from build123d import *

# Parameters (mm, degrees)
F0_W     = 50.8
F0_H     = 50.8
F0_W_2   = 41.275
F0_H_2   = 41.275
F1_DEPTH = 171.45
F2_R     = 5.08
F3_R     = 5.08


with BuildPart() as f1:
    # F0 (on Front) → F1 (new body, symmetric)
    with BuildSketch(Plane.XZ):
        Rectangle(F0_W, F0_H)
        Rectangle(F0_W_2, F0_H_2, mode=Mode.SUBTRACT)
    extrude(amount=F1_DEPTH, both=True)

    # F2
    f2_edges = [f1.edges().sort_by_distance(p)[0] for p in [
        (-20.6375, 0, 20.6375),
        (-25.4, 0, -25.4),
        (25.4, 0, -25.4),
        (20.6375, 0, 20.6375),
        (25.4, 0, 25.4),
        (-25.4, 0, 25.4),
    ]]
    fillet(f2_edges, radius=F2_R)

    # F3
    f3_edges = [f1.edges().sort_by_distance(p)[0] for p in [
        (-20.6375, 0, -20.6375),
        (20.6375, 0, -20.6375),
    ]]
    fillet(f3_edges, radius=F3_R)


solid = f1.part
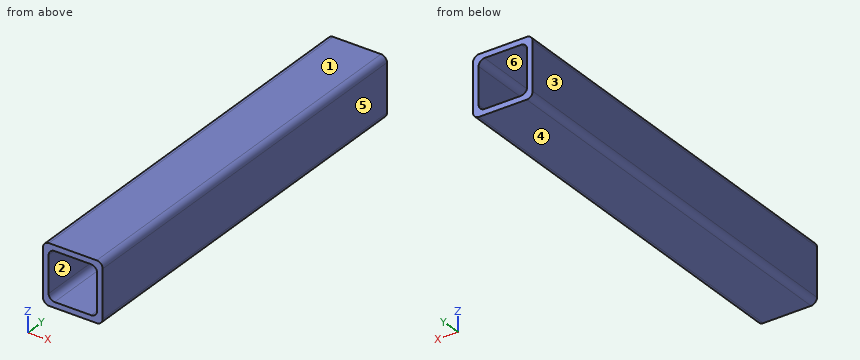
Geometry: final body of the model. Coordinates: model frame, mm. Face numbers are marked on the shaded views. A direction names the side the tool comes from. Give positions to 0.01 mm unless a question says otherwise; leave off trailing zeros. Write each loop counter-clockwise with the first axis right and the second up, starting at its lowest first coordinate (ties: lowest second). Pieces come first, ordered by that corner, then holes. Notation, with made-up numbers: (8.25, 67) - (43.25, 67) arc R13 ccw to (43.25, 89) - close; hole circle Ø2 at (30, 87.25). An arc over 180 degrees is marked (long way). Return JSON: item names as keys, results as strings. Group by question number.
1) Set-up query: the marked faces 5 and 6. Return all of +Z, -Z, +X, -X, +Y, -Y with unobstructed straight access to the full face (end or side cutting, diameter ignored); none if empty.
2) First-contact query: P1, Ø2, axis at x = -18.5, z = -16, coming from the -Y side. Flat tip, straight axial feed; report the tip coordinate or a pass-through.
3) Section A-A on x = -3. Return the cut outline in (y, z).
4) Line query: line 1 (Z direction, x = 2, y = -0.5); line 2 (X direction, y = 56, z = -21). Output: solid intervals per line, ascending.
5) Section B-B on z = 2. Return the cut outline in (x, y), plus the area to 3 significant figures.
6) Mould query, pull axis Z, two halves, no side actions, for the marked faces 1, 2, 3 and 4. Classes: released by +Z, released by -Z, zero draft, split by the parting line, or undercut.
7) Section C-C on y = 70. Return the cut outline in (x, z).
Filled in:
{
 "1": {"face 5": "+Z, -Z, +X, +Y, -Y", "face 6": "+Y, -Y"},
 "2": {"P1": "passes through"},
 "3": {"outline": "(-171.45, -25.4) - (171.45, -25.4) - (171.45, -20.64) - (-171.45, -20.64) - close; (-171.45, 20.64) - (171.45, 20.64) - (171.45, 25.4) - (-171.45, 25.4) - close"},
 "4": {"line 1": "z = -25.4 to -20.64, 20.64 to 25.4", "line 2": "x = -25.35 to 25.35"},
 "5": {"outline": "(-25.4, -171.45) - (-20.64, -171.45) - (-20.64, 171.45) - (-25.4, 171.45) - close; (20.64, -171.45) - (25.4, -171.45) - (25.4, 171.45) - (20.64, 171.45) - close", "area": "3,270 mm^2"},
 "6": {"face 1": "released by +Z", "face 2": "undercut", "face 3": "zero draft", "face 4": "released by -Z"},
 "7": {"outline": "(-25.4, -20.32) arc R5.08 ccw to (-20.32, -25.4) - (20.32, -25.4) arc R5.08 ccw to (25.4, -20.32) - (25.4, 20.32) arc R5.08 ccw to (20.32, 25.4) - (-20.32, 25.4) arc R5.08 ccw to (-25.4, 20.32) - close; hole (-20.64, -15.56) arc R5.08 ccw to (-15.56, -20.64) - (15.56, -20.64) arc R5.08 ccw to (20.64, -15.56) - (20.64, 15.56) arc R5.08 ccw to (15.56, 20.64) - (-15.56, 20.64) arc R5.08 ccw to (-20.64, 15.56) - close"}
}
